Source: three-view drawing plus pictorial views. Frame: mm from the lowest corner of the part. A direction names the side the tool comes from. Give positions to 0.01 mm unless a question says otherwise; leave off trailing zeros. Write each loop counter-clockwise with the first axis right and the second up, starting at its lowest first coordinate (ties: lowest second). Pieces come first, ordered by that corner, then holes. Notation, with made-up numbers: (-12.5, 33) -> (33.5, 33) arc R9 cw to (33.5, 45) -> close; hole circle Ø6 at (30, 24.25). An arc over 180 degrees is marked (long way). Write item = value, one per line.
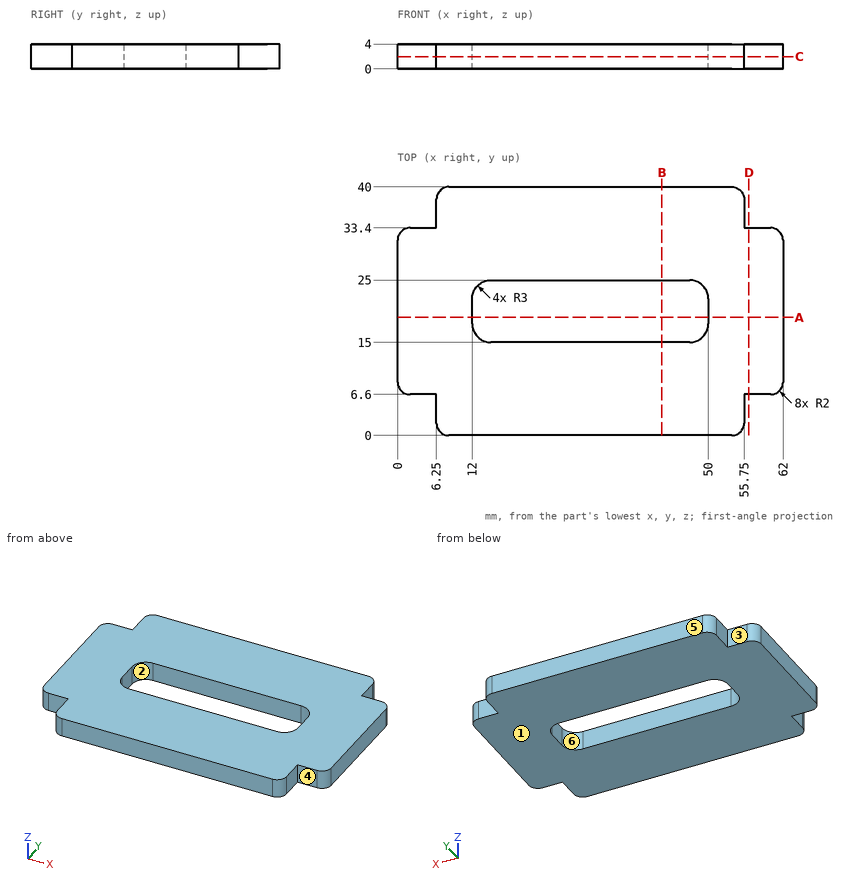
1) Contact query for flat-ended pins moving along their axis: pin 1 (1.2 mm diameter, centred on y = 21, z = 1.5, fed in from -X); pin 2 (2 mm diameter, centred on y = 36, z = 1, fed in from -X); pin 3 (1.2 mm diameter, centred on y = 5, z = 2.5, fed in from +X); pin 4 (2 mm diameter, centred on x = 3.5, z = 2.5, fed in from +Y). Output: stop coordinate, or through.
Computed:
pin_1 = 0
pin_2 = 6.25
pin_3 = 55.75
pin_4 = 33.4
2) Cut plane D-D (x = 56.5). Return the cut outline in (y, z).
Computed:
outline = (6.6, 0) -> (33.4, 0) -> (33.4, 4) -> (6.6, 4) -> close
3) Access query for the marked faces 4, 5 and 6. Directions: +Z, -Z, +X, -X, +Y, -Y. A direction counts if a zero-diameter tool reaches every point of the face in a straight line with its end or side. Return the directions, or none.
Computed:
face_4 = +Z, -Z, +X, -Y
face_5 = +Z, -Z, +X, -X, +Y
face_6 = +Z, -Z
4) Material intervals for L1, parallel to X at y = 18.5, z = 3.35; L2, parallel to Y at x = 16, z = 1.35; L3, parallel to Y at x = 6, z = 0.65, sorted ascending.
Computed:
L1 = 0 to 12, 50 to 62
L2 = 0 to 15, 25 to 40
L3 = 6.6 to 33.4
5) Cut plane A-A (y = 19). Return the cut outline in (x, z), then the cut area to 3 significant figures.
Computed:
outline = (0, 0) -> (12, 0) -> (12, 4) -> (0, 4) -> close; (50, 0) -> (62, 0) -> (62, 4) -> (50, 4) -> close
area = 96.0 mm²
6) Draft query along Y for the marked faces 1, 2 and 3. Return one class per face: pulls with the +Y half, pulls with the -Y half, needs draft (parallel to the pull), parting line crosses it, or undercut.
Computed:
face_1 = needs draft
face_2 = undercut
face_3 = pulls with the +Y half
7) Cut plane C-C (z = 1.95). Return the cut outline in (x, y).
Computed:
outline = (0, 8.6) arc R2 ccw to (2, 6.6) -> (6.25, 6.6) -> (6.25, 2) arc R2 ccw to (8.25, 0) -> (53.75, 0) arc R2 ccw to (55.75, 2) -> (55.75, 6.6) -> (60, 6.6) arc R2 ccw to (62, 8.6) -> (62, 31.4) arc R2 ccw to (60, 33.4) -> (55.75, 33.4) -> (55.75, 38) arc R2 ccw to (53.75, 40) -> (8.25, 40) arc R2 ccw to (6.25, 38) -> (6.25, 33.4) -> (2, 33.4) arc R2 ccw to (0, 31.4) -> close; hole (12, 18) arc R3 ccw to (15, 15) -> (47, 15) arc R3 ccw to (50, 18) -> (50, 22) arc R3 ccw to (47, 25) -> (15, 25) arc R3 ccw to (12, 22) -> close
8) Cut plane B-B (x = 42.5). Return the cut outline in (y, z).
Computed:
outline = (0, 0) -> (15, 0) -> (15, 4) -> (0, 4) -> close; (25, 0) -> (40, 0) -> (40, 4) -> (25, 4) -> close
